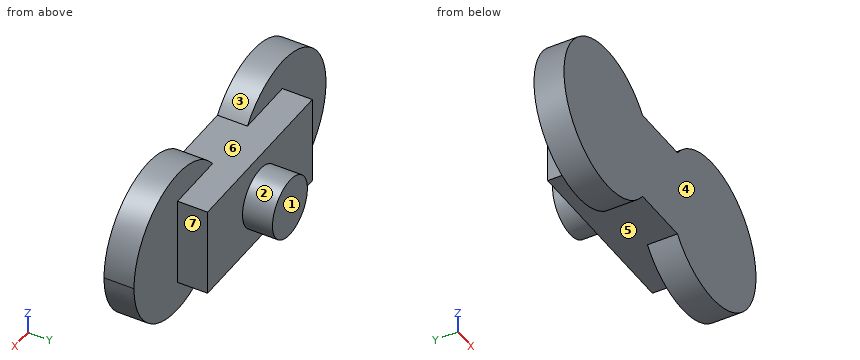
```python
from build123d import *

# Parameters (mm, degrees)
EXTRUDE_1_DEPTH   = 10
EXTRUDE_1_2_DEPTH = 10
EXTRUDE_2_DEPTH   = 20
SKETCH_7_R        = 10
EXTRUDE_4_DEPTH   = 30


with BuildPart() as part:
    # Sketch 1 → Extrude 1 (new body)
    with BuildSketch(Plane(origin=(0, 0, 0), x_dir=(1, 0, 0), z_dir=(0, 1, 0))):
        with BuildLine():
            Line((20.689216343, -8.628600134), (20.689216343, -38.628600134))
            Line((20.689216343, -38.628600134), (0.689216343, -38.628600134))
            ThreePointArc((0.689216343, -38.628600134), (28.594910493, -47.345682585), (45.689216343, -23.628600134))
            ThreePointArc((45.689216343, -23.628600134), (28.594910493, 0.088482317), (0.689216343, -8.628600134))
            Line((0.689216343, -8.628600134), (20.689216343, -8.628600134))
        make_face()
    extrude(amount=EXTRUDE_1_DEPTH)



with BuildPart() as body_2:
    # Sketch 1 → Extrude 1 2 (new body)
    with BuildSketch(Plane(origin=(0, 0, 0), x_dir=(1, 0, 0), z_dir=(0, 1, 0))):
        with BuildLine():
            ThreePointArc((-19.310783657, -8.628600134), (-64.310783657, -23.628600134), (-19.310783657, -38.628600134))
            Line((-19.310783657, -38.628600134), (-39.310783657, -38.628600134))
            Line((-39.310783657, -38.628600134), (-39.310783657, -8.628600134))
            Line((-39.310783657, -8.628600134), (-19.310783657, -8.628600134))
        make_face()
    extrude(amount=EXTRUDE_1_2_DEPTH)


with BuildPart() as part_1:
    add(part.part)

    add(body_2.part)  # Extrude 2 merges body 2
    # Sketch 1_3 → Extrude 2 (add)
    with BuildSketch(Plane(origin=(0, 0, 0), x_dir=(1, 0, 0), z_dir=(0, 1, 0))):
        with BuildLine():
            Line((0.689216343, -38.628600134), (20.689216343, -38.628600134))
            Line((20.689216343, -38.628600134), (20.689216343, -8.628600134))
            Line((20.689216343, -8.628600134), (0.689216343, -8.628600134))
            ThreePointArc((0.689216343, -8.628600134), (-1.479526151, -12.072352636), (-3.060783657, -15.822352636))
            ThreePointArc((-3.060783657, -15.822352636), (-0.296905468, -19.298473115), (0.689216343, -23.628600134))
            ThreePointArc((0.689216343, -23.628600134), (-0.296905468, -27.958727153), (-3.060783657, -31.434847632))
            ThreePointArc((-3.060783657, -31.434847632), (-1.479526151, -35.184847632), (0.689216343, -38.628600134))
        make_face()
        with BuildLine():
            ThreePointArc((-3.060783657, -15.822352636), (-1.479526151, -12.072352636), (0.689216343, -8.628600134))
            Line((0.689216343, -8.628600134), (-19.310783657, -8.628600134))
            ThreePointArc((-19.310783657, -8.628600134), (-17.142041163, -12.072352636), (-15.560783657, -15.822352636))
            ThreePointArc((-15.560783657, -15.822352636), (-9.310783657, -13.628600134), (-3.060783657, -15.822352636))
        make_face()
        with BuildLine():
            Line((-19.310783657, -38.628600134), (0.689216343, -38.628600134))
            ThreePointArc((0.689216343, -38.628600134), (-1.479526151, -35.184847632), (-3.060783657, -31.434847632))
            ThreePointArc((-3.060783657, -31.434847632), (-9.310783657, -33.628600134), (-15.560783657, -31.434847632))
            ThreePointArc((-15.560783657, -31.434847632), (-17.142041163, -35.184847632), (-19.310783657, -38.628600134))
        make_face()
        with BuildLine():
            Line((-39.310783657, -38.628600134), (-19.310783657, -38.628600134))
            ThreePointArc((-19.310783657, -38.628600134), (-17.142041163, -35.184847632), (-15.560783657, -31.434847632))
            ThreePointArc((-15.560783657, -31.434847632), (-19.310783657, -23.628600134), (-15.560783657, -15.822352636))
            ThreePointArc((-15.560783657, -15.822352636), (-17.142041163, -12.072352636), (-19.310783657, -8.628600134))
            Line((-19.310783657, -8.628600134), (-39.310783657, -8.628600134))
            Line((-39.310783657, -8.628600134), (-39.310783657, -38.628600134))
        make_face()
    extrude(amount=EXTRUDE_2_DEPTH)

    # Sketch 7 → Extrude 4 (add)
    with BuildSketch(Plane.XZ):
        with Locations(Location((-9.310783657, 23.628600134, 0), (0, 0, 270))):
            Circle(SKETCH_7_R)
    extrude(amount=-EXTRUDE_4_DEPTH)


solid = part_1.part
```
The model under review builds one solid part; all positions refer to its coordinate system, in mm. Face numbers are marked on the shaded views. A direction names the side the tool comes from. Round coordinates to 2 decimals unless told otherwise and drop trailing zeros. Loops run counter-clockwise (first coordinate to the right, second up) from the corner with the lowest first, then second, coordinate; pieces in that order, holes last.
1) Consider section C-C on z = 4.5. State the section outline as (x, y) points, then the cut area to 3 significant figures.
Values follow:
outline: (-55.41, 0) - (-23.21, 0) - (-23.21, 10) - (-55.41, 10) - close; (4.59, 0) - (36.79, 0) - (36.79, 10) - (4.59, 10) - close
area: 644 mm2
2) Consider section D-D on z = 20.5. State the section outline as (x, y) points, then the cut area to 3 significant figures.
Values follow:
outline: (-64.11, 0) - (45.49, 0) - (45.49, 10) - (20.69, 10) - (20.69, 20) - (0.19, 20) - (0.19, 30) - (-18.81, 30) - (-18.81, 20) - (-39.31, 20) - (-39.31, 10) - (-64.11, 10) - close
area: 1,890 mm2
3) Consider section A-A on y = 5.5. State the section outline as (x, z) points.
Values follow:
outline: (-19.31, 8.63) - (0.69, 8.63) arc R25 ccw (long way) to (0.69, 38.63) - (-19.31, 38.63) arc R25 ccw (long way) to start
4) Wall thickness on line 1 along X through (y, z) = (15.75, 22); line 2 along Y through (x, z) = (21, 14); line 3 along Y through (x, z) = (-14.5, 33.5): over which ranges is each line inside the solid? List them lowest first.
Values follow:
line 1: x = -39.31 to 20.69
line 2: y = 0 to 10
line 3: y = 0 to 20
5) Consider section B-B on x = -31. State the section outline as (y, z) points.
Values follow:
outline: (0, 0.05) - (10, 0.05) - (10, 8.63) - (20, 8.63) - (20, 38.63) - (10, 38.63) - (10, 47.21) - (0, 47.21) - close
6) Tool access review of the marked faces 4, 5, 6 and 7: name each direction out of +Z, -Z, +X, -X, +Y, -Y from which nothing blocks a thin tool from reaching the whole face with its end or side.
Values follow:
face 4: +Z, -Z, +X, -X, -Y
face 5: -Z, +Y
face 6: +Z, +Y
face 7: +Z, -Z, +X, +Y
7) Clearance check with flat-ended pins moving along their axes: P1, Ø12, axis at x = 32, y = 12, coming from the +Z side; P2, Ø5, axis at y = 13, z = 26.5, coming from the +X side; P3, Ø12, axis at x = 27, z = 26.5, coming from the -Y side; P4, Ø8, axis at y = 8, z = 4, coming from the -X side. State where each tip first meets the part, or that it passes through.
Values follow:
P1: stops at z = 47.98
P2: stops at x = 20.69
P3: stops at y = 0
P4: stops at x = -58.82
8) The part is to be moulded in two halves that separate along X. For the marked faces 1, 2 and 3, say which applies: pulls with the +X half, pulls with the -X half, needs draft (parallel to the pull), parting line crosses it, or undercut.
Values follow:
face 1: needs draft
face 2: parting line crosses it
face 3: undercut
